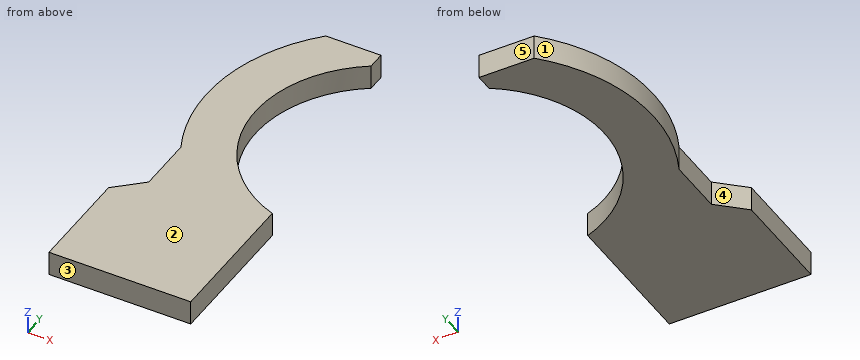
from build123d import *

# Parameters (mm, degrees)
CYLINDER002_R     = 0.5
CYLINDER002_DEPTH = 15
PAD001_DEPTH      = 7


with BuildPart() as fixation_servo:
    # Cylinder002 → Cylinder002 (new body)
    with BuildSketch(Plane(origin=(38, 30, 0), x_dir=(1, 0, 0), z_dir=(0, 0, 1))):
        Circle(CYLINDER002_R)
    extrude(amount=CYLINDER002_DEPTH)


with BuildPart() as part_mirroring001:
    # Part__Mirroring001: instance of fixation_servo
    add(fixation_servo.part.mirror(Plane(origin=(0, 0, 0), x_dir=(0, -1, 0), z_dir=(1, 0, 0))))


with BuildPart() as cut004:
    # Sketch001 → Pad001 (new body)
    with BuildSketch(Plane.XY):
        with BuildLine():
            Line((20.522763, 10), (-20, 10))
            Line((-20, 10), (-20, 40))
            Line((-20, 40), (-12.44178, 46.907085))
            Line((-12.44178, 63.085703), (-12.44178, 46.907085))
            ThreePointArc((-3.272439, 119.933259), (-16.862004, 92.961944), (-12.44178, 63.085703))
            Line((12.5, 119.933259), (-3.272439, 119.933259))
            Line((12.5, 119.933259), (12.5, 114.933259))
            ThreePointArc((12.5, 114.933259), (-3.21942, 80.514127), (20.522763, 51.050835))
            Line((20.522763, 51.050835), (20.522763, 10))
        make_face()
    extrude(amount=PAD001_DEPTH)

    # Cut004: cut Part__Mirroring001
    add(part_mirroring001.part, mode=Mode.SUBTRACT)


solid = cut004.part
Geometry: final body of the model. Coordinates: model frame, mm. Face numbers are marked on the shaded views. A direction names the side the tool comes from. Round coordinates to 2 decimals unless told otherwise and drop trailing zeros. Loops run counter-clockwise (first coordinate to the right, second up) from the corner with the lowest first, then second, coordinate; pieces in that order, holes last. Notation, with made-up numbers: M -31,59 L -26,59 A36 cw -26,97 Z; hole C 6,31 d7. An arc over 180 degrees is marked long. Put each result on its own line as item: value. Start each with the question number.
(1) Set-up query: the marked faces 4 and 5. Return all of +Z, -Z, +X, -X, +Y, -Y with unobstructed straight access to the full face (end or side cutting, diameter ignored); none if empty.
(2) Section query A-A (x = 5). Return loops of the section in (y, z), then the cut area to 3 significant figures.
(3) Contact query for flat-ended pins moving along their axis: pin 1 Ø4 at (y, z) = (117, 3) entering from +X; pin 2 Ø3 at (y, z) = (82.5, 1.5) entering from -X; pin 3 Ø1.5 at (x, z) = (-11, 1) entering from +Y. Output: stop coordinate, or through.
(4) Section query B-B (z = 3.75). Return loops of the section in (x, y), then the cut area to 3 significant figures.
(5) Section query D-D (y = 99.5). Return loops of the section in (x, z).
(6) Material intervals for line 1 along X through (y, z) = (48.5, 0.5); line 2 along Y through (x, z) = (-0.5, 4); line 3 along X through (y, z) = (84, 6.25), sorted ascending. Write a range as [from, to].
(7) Section query C-C (x = -2). Return loops of the section in (y, z).
(8) Draft query along Y for the marked faces 1, 2 and 3. Return one class per face: +Y half, -Y half, draft (parallel to the pull), parting line (faces both ways), or undercut.
Findings below:
1. face 4: +Z, -Z, -X
1. face 5: +Z, -Z, +X, -X, +Y
2. outline: M 10,0 L 61.77,0 L 61.77,7 L 10,7 Z; M 108.23,0 L 119.93,0 L 119.93,7 L 108.23,7 Z
2. area: 444 mm2
3. pin 1: stops at x = 12.5
3. pin 2: stops at x = -17.49
3. pin 3: stops at y = 110.93
4. outline: M -20,10 L 20.52,10 L 20.52,51.05 A36 cw 12.5,114.93 L 12.5,119.93 L -3.27,119.93 A50 ccw -12.44,63.09 L -12.44,46.91 L -20,40 Z
4. area: 2,760 mm2
5. outline: M -15.35,0 L -0.45,0 L -0.45,7 L -15.35,7 Z
6. line 1: x = [-12.44, 20.52]
6. line 2: y = [10, 70.61], [99.39, 119.93]
6. line 3: x = [-17.49, -3.49]
7. outline: M 10,0 L 74.72,0 L 74.72,7 L 10,7 Z; M 95.28,0 L 119.93,0 L 119.93,7 L 95.28,7 Z
8. face 1: undercut
8. face 2: draft
8. face 3: -Y half
